Part print with two shaded views. Sizes in mm from the minimum x, y, z corner. Round coordinates to 2 decimals unless told otherwise and drop trailing zeros. Write each loop counter-clockwise with the first axis right and the second up, starting at its lowest first coordinate (ties: lowest second). Pieces come first, ordered by that corner, then holes. Notation, with made-up numbers: (-14.5, 19) -> (-6.5, 19) arc R19 cw to (-6.5, 40) -> close; hole circle Ø2 at (61.5, 4.25). An arc over 180 degrees is marked (long way). Answer in a Markdown table with one row per item.
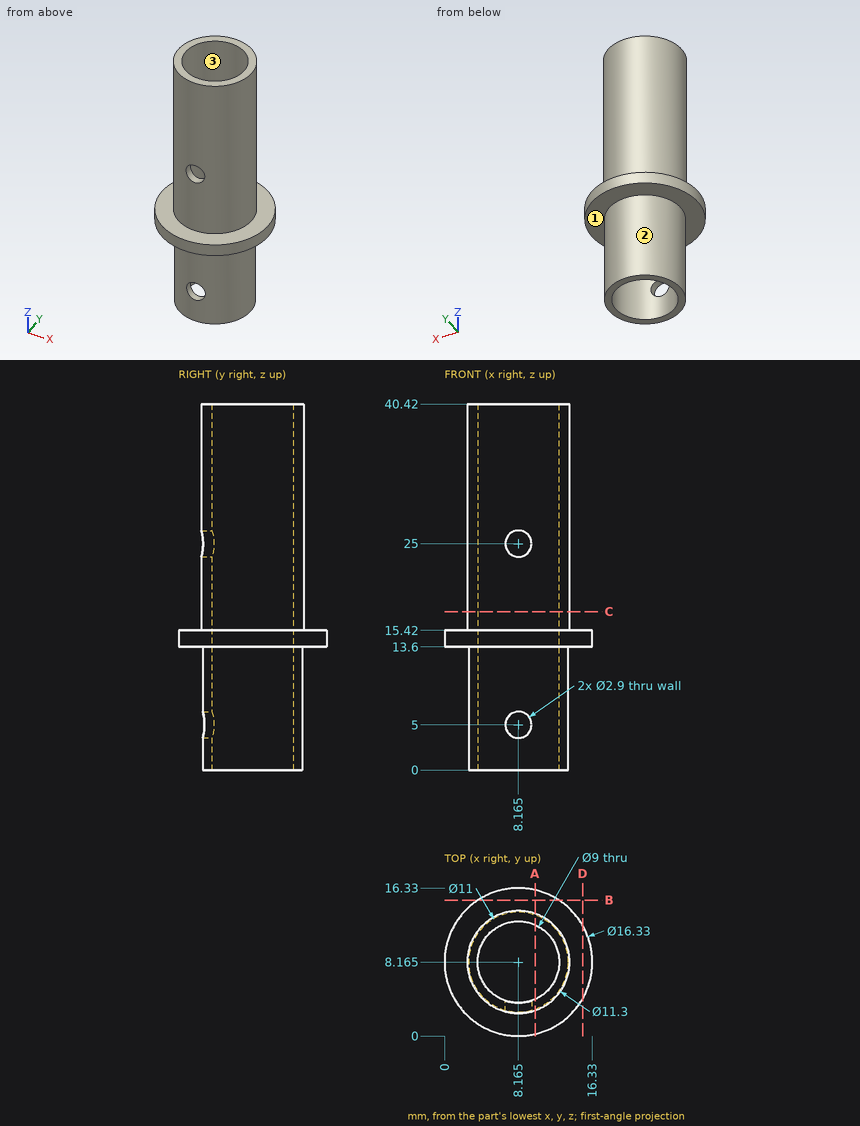
Q1. Saw through at D-D on x = 15.25. Write the cut outline in (y, z), plus the area to 3 significant figures.
A:
| item | result |
|---|---|
| outline | (4.11, 13.6) -> (12.22, 13.6) -> (12.22, 15.42) -> (4.11, 15.42) -> close |
| area | 14.8 mm² |
Q2. Saw through at A-A on x = 10. Write the cut outline in (y, z).
A:
| item | result |
|---|---|
| outline | (0.21, 13.6) -> (2.98, 13.6) -> (2.98, 0) -> (4.06, 0) -> (4.06, 40.42) -> (2.82, 40.42) -> (2.82, 15.42) -> (0.21, 15.42) -> close; (12.27, 0) -> (13.35, 0) -> (13.35, 13.6) -> (16.12, 13.6) -> (16.12, 15.42) -> (13.51, 15.42) -> (13.51, 40.42) -> (12.27, 40.42) -> close |
Q3. Wall check: line 1 (Z direction, x = 1, y = 11.25); line 2 (Y direction, x = 11.75, z = 19); line 3 (Y direction, x = 9, z = 22.5). Give the ranges that are in metal, low to high. Write a range as [from, to].
A:
| item | result |
|---|---|
| line 1 | [13.6, 15.42] |
| line 2 | [3.8, 5.45], [10.88, 12.53] |
| line 3 | [2.58, 3.74], [12.59, 13.75] |
Q4. Two-plate mould, pull along X, no slides. Class the marked faces 1, 2 and 3: released by +X, released by -X, zero draft, split by the parting line, or undercut.
A:
| item | result |
|---|---|
| face 1 | zero draft |
| face 2 | split by the parting line |
| face 3 | undercut |
Q5. Saw through at C-C on z = 17.5. Write the cut outline in (x, y) (3 decimals).
A:
| item | result |
|---|---|
| outline | circle Ø11.3 at (8.165, 8.165); hole circle Ø9 at (8.165, 8.165) |
Q6. Drop flat-ended pins along their axis: P1, Ø8, axis at x = 5, y = 6, coming from the +Z side; P2, Ø4, axis at x = 8.165, z = 25, coming from the -Y side (3 decimals); P3, Ø4, axis at y = 14.5, z = 7, coming from the -X side; P4, Ø8, axis at x = 5.5, z = 30.5, coming from the +Y side (3 decimals). Give the stop position or say it passes through.
A:
| item | result |
|---|---|
| P1 | z = 40.42 |
| P2 | y = 2.515 |
| P3 | x = 4.78 |
| P4 | y = 13.815 |
Q7. Saw through at B-B on y = 15. Write the cut outline in (x, z).
A:
| item | result |
|---|---|
| outline | (3.7, 13.6) -> (12.63, 13.6) -> (12.63, 15.42) -> (3.7, 15.42) -> close |
